Design review of the part built by this model. Coordinates are the model's own, in mm. Face numbers are marked on the shaded views. A direction names the side the tool comes from. Give positions to 0.01 mm unless a question says otherwise; leave off trailing zeros. Write each loop counter-clockwise with the first axis right and the second up, starting at its lowest first coordinate (ties: lowest second). Pieces come first, ordered by that corner, then holes.
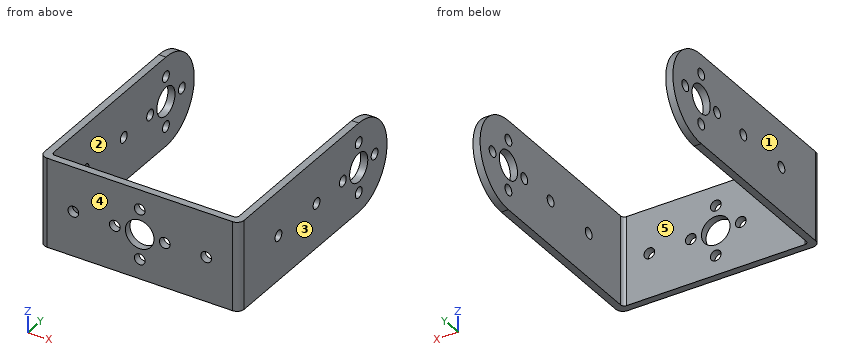
```python
from build123d import *

# Parameters (mm, degrees)
EXTRUDE_1_DEPTH           = 56
SKETCH_2_W                = 52
SKETCH_2_H                = 100
CUT_EXTRUDE_1_DEPTH       = 88.562834582
HOLE_WIZARD_8_0_8_1_D     = 8
HOLE_WIZARD_8_0_8_1_DEPTH = 2
HOLE_WIZARD_8_0_8_2_D     = 8
HOLE_WIZARD_3_0_3_1_D     = 3
HOLE_WIZARD_3_0_3_1_DEPTH = 2
HOLE_WIZARD_3_0_3_2_D     = 3
HOLE_WIZARD_3_0_3_3_D     = 3
HOLE_WIZARD_8_0_8_3_D     = 8
FILLET_1_R                = 1
FILLET_2_R                = 2


with BuildPart() as part:
    # 草图1 → 凸台-拉伸1 (new body)
    with BuildSketch(Plane(origin=(56, 0, 0), x_dir=(0, 0, -1), z_dir=(1, 0, 0))):
        with BuildLine():
            Line((-25, 50), (-25, -2.5))
            Line((-25, -2.5), (0, -2.5))
            Line((0, -2.5), (0, 50))
            ThreePointArc((0, 50), (-12.5, 62.5), (-25, 50))
        make_face()
    extrude(amount=-EXTRUDE_1_DEPTH)

    # 草图2 → 切除-拉伸1 (cut, through all)
    with BuildSketch(Plane.XY.offset(25)):
        with Locations((28, 49.5)):
            Rectangle(SKETCH_2_W, SKETCH_2_H)
    extrude(amount=-CUT_EXTRUDE_1_DEPTH, mode=Mode.SUBTRACT)

    # Ø8.0 (8) 直径孔1
    with Locations(Plane(origin=(56, 0, 0), x_dir=(0, 0, -1), z_dir=(1, 0, 0))):
        with Locations((-12.5, 50)):
            Hole(HOLE_WIZARD_8_0_8_1_D / 2, depth=HOLE_WIZARD_8_0_8_1_DEPTH)

    # Ø8.0 (8) 直径孔2 (through all)
    with Locations(Plane(origin=(2, 0, 0), x_dir=(0, 0, -1), z_dir=(1, 0, 0))):
        with Locations((-12.5, 50)):
            Hole(HOLE_WIZARD_8_0_8_2_D / 2)

    # Ø3.0 (3) 直径孔1
    with Locations(Plane(origin=(56, 0, 0), x_dir=(0, 0, -1), z_dir=(1, 0, 0))):
        with Locations((-5.5, 50), (-12.5, 57), (-12.5, 31.4), (-12.5, 43), (-19.5, 50), (-12.5, 14.6)):
            Hole(HOLE_WIZARD_3_0_3_1_D / 2, depth=HOLE_WIZARD_3_0_3_1_DEPTH)

    # Ø3.0 (3) 直径孔2 (through all)
    with Locations(Plane(origin=(2, 0, 0), x_dir=(0, 0, -1), z_dir=(1, 0, 0))):
        with Locations((-5.5, 50), (-12.5, 57), (-12.5, 31.4), (-12.5, 43), (-19.5, 50), (-12.5, 14.6)):
            Hole(HOLE_WIZARD_3_0_3_2_D / 2)

    # Ø3.0 (3) 直径孔3 (through all)
    with Locations(Plane(origin=(0, -2.5, 0), x_dir=(-1, 0, 0), z_dir=(0, -1, 0))):
        with Locations((-46.6, -12.5), (-21, -12.5), (-35, -12.5), (-9.4, -12.5), (-28, -19.5), (-28, -5.5)):
            Hole(HOLE_WIZARD_3_0_3_3_D / 2)

    # Ø8.0 (8) 直径孔3 (through all)
    with Locations(Plane(origin=(0, -2.5, 0), x_dir=(-1, 0, 0), z_dir=(0, -1, 0))):
        with Locations((-28, -12.5)):
            Hole(HOLE_WIZARD_8_0_8_3_D / 2)

    # 圆角1
    fillet_1_edges = [part.edges().sort_by_distance(p)[0] for p in [
        (54, -0.5, 12.5),
        (2, -0.5, 12.5),
    ]]
    fillet(fillet_1_edges, radius=FILLET_1_R)

    # 圆角2
    fillet_2_edges = [part.edges().sort_by_distance(p)[0] for p in [
        (0, -2.5, 12.5),
        (56, -2.5, 12.5),
    ]]
    fillet(fillet_2_edges, radius=FILLET_2_R)


solid = part.part
```
(1) To check wall thickness, follow L1, parallel to X at y = 44.5, z = 10.25; L2, parallel to Z at x = 21, y = -1.6; L3, parallel to Y at x = 47.5, z = 2. State the ranges of each line that lie inside material, in increasing order.
Resolved:
L1: x = 0 to 2, 54 to 56
L2: z = 0 to 11, 14 to 25
L3: y = -2.5 to -0.5
(2) Tool access review of the marked faces 1 and 2: name each direction out of +Z, -Z, +X, -X, +Y, -Y from which nothing blocks a thin tool from reaching the whole face with its end or side.
Resolved:
face 1: +Z, -Z, -X, +Y, -Y
face 2: +Z, -Z, +Y
(3) Consider section B-B, the plane y = 31.4. Give the boundary of the cut face in (x, z), then the cut area to 3 significant figures.
Resolved:
outline: (0, 0) - (2, 0) - (2, 11) - (0, 11) - close; (0, 14) - (2, 14) - (2, 25) - (0, 25) - close; (54, 0) - (56, 0) - (56, 11) - (54, 11) - close; (54, 14) - (56, 14) - (56, 25) - (54, 25) - close
area: 88.0 mm2
(4) Consider section A-A, the plane x = 21. Give the boundary of the cut face in (y, z).
Resolved:
outline: (-2.5, 0) - (-0.5, 0) - (-0.5, 11) - (-2.5, 11) - close; (-2.5, 14) - (-0.5, 14) - (-0.5, 25) - (-2.5, 25) - close
(5) Consider section C-C, the plane x = 28. Give the boundary of the cut face in (y, z), then the cut area to 3 significant figures.
Resolved:
outline: (-2.5, 0) - (-0.5, 0) - (-0.5, 4) - (-2.5, 4) - close; (-2.5, 7) - (-0.5, 7) - (-0.5, 8.5) - (-2.5, 8.5) - close; (-2.5, 16.5) - (-0.5, 16.5) - (-0.5, 18) - (-2.5, 18) - close; (-2.5, 21) - (-0.5, 21) - (-0.5, 25) - (-2.5, 25) - close
area: 22.0 mm2
(6) Consider section D-D, the plane z = 5.5. Give the boundary of the cut face in (x, y).
Resolved:
outline: (0, -0.5) arc R2 ccw to (2, -2.5) - (26.5, -2.5) - (26.5, -0.5) - (3, -0.5) arc R1 cw to (2, 0.5) - (2, 48.5) - (0, 48.5) - close; (0, 51.5) - (2, 51.5) - (2, 60.36) - (0, 60.36) - close; (29.5, -2.5) - (54, -2.5) arc R2 ccw to (56, -0.5) - (56, 48.5) - (54, 48.5) - (54, 0.5) arc R1 cw to (53, -0.5) - (29.5, -0.5) - close; (54, 51.5) - (56, 51.5) - (56, 60.36) - (54, 60.36) - close
(7) Clearance check with a flat-ended pin moving along its axis: P1, Ø1.5, axis at x = 18, z = 15, coming from the +Y side. State where the tip first meets the part, or that it passes through.
Resolved:
P1: stops at y = -0.5
(8) Mouldability with a two-part tool opening along X and no side actions: class the marked faces 3, 4 and 5 as pulls with the +X half, pulls with the -X half, needs draft (parallel to the pull), parting line crosses it, or undercut.
Resolved:
face 3: pulls with the +X half
face 4: needs draft
face 5: undercut
